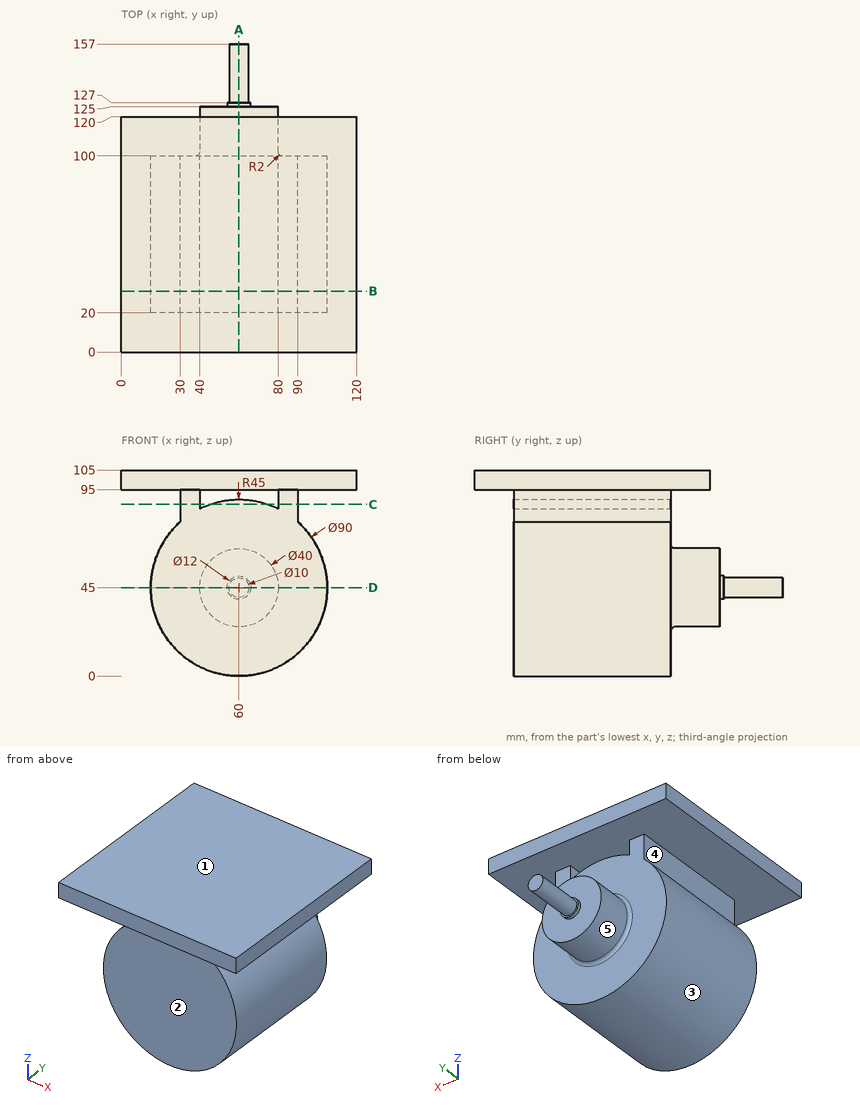
Answer from the drawing. Dimensions are ordinates in mm from the lowest x, y and z of the part. A direction names the side the tool comes from. Give positions to 0.01 mm unless a question says otherwise; leave off trailing zeros. Write each loop counter-clockwise with the first axis right and the second up, starting at its lowest first coordinate (ties: lowest second). Pieces come first, ordered by that corner, then holes. Notation, with made-up numbers: (32.25, -18) - (80.25, -18) arc R11 ccw to (80.25, -9) - close; hole circle Ø2 at (48, -15). An arc over 180 degrees is marked (long way). Answer in a Markdown table with one row per item. Add a question column.
Item 1: Find the intervals of material crossed by L1, parallel to X at y = 88, z = 43.5 (3 decimals); L2, parallel to Z at x = 93.5, y = 11; L3, parallel to Y at x = 30, z = 35.5, in increasing order.
Item 2: Section A-A, the plane x = 60 is taken. Write down the section's boundary in (y, z).
Item 3: Section D-D, the plane z = 45 is taken. Write down the section's boundary in (x, y).
Item 4: Determine the mould class of the marked faces 1, 2 and 3 for opening direction Z: pulls with the +Z half, pulls with the -Z half, needs draft (parallel to the pull), parting line crosses it, or undercut.
Item 5: Section B-B, the plane y = 31 is taken. Write down the section's boundary in (x, z).
Item 6: Flat-ended cylindrical pins translate along their axes: P1, Ø1.5, axis at x = 90.5, y = 74, coming from the -Z side; P2, Ø5, axis at y = 67, z = 90.5, coming from the +X side; P3, Ø1, axis at x = 82.5, z = 16.5, coming from the -Y side. Find the tip coordinate at first contact, or state that the pin passes through.
Item 7: A tool of negligible diameter and unlimited length cuts with its end or side. For the marked faces 4 and 5, from which of +Z, -Z, +X, -X, +Y, -Y can it reach the whole face along a straight path? Write none if from no direction.
Item 8: Section C-C, the plane z = 87.5 is taken. Write down the section's boundary in (x, y).
Recorded:
| question | item | result |
|---|---|---|
| 1 | L1 | x = 15.025 to 104.975 |
| 1 | L2 | z = 95 to 105 |
| 1 | L3 | y = 20 to 100 |
| 2 | outline | (0, 95) - (120, 95) - (120, 105) - (0, 105) - close; (20, 0) - (100, 0) - (100, 23) arc R2 cw to (102, 25) - (125, 25) - (125, 39) - (127, 39) - (127, 40) - (157, 40) - (157, 50) - (127, 50) - (127, 51) - (125, 51) - (125, 65) - (102, 65) arc R2 cw to (100, 67) - (100, 90) - (20, 90) - close |
| 3 | outline | (15, 20) - (105, 20) - (105, 100) - (82, 100) arc R2 cw to (80, 102) - (80, 125) - (66, 125) - (66, 127) - (65, 127) - (65, 157) - (55, 157) - (55, 127) - (54, 127) - (54, 125) - (40, 125) - (40, 102) arc R2 cw to (38, 100) - (15, 100) - close |
| 4 | face 1 | pulls with the +Z half |
| 4 | face 2 | needs draft |
| 4 | face 3 | undercut |
| 5 | outline | (0, 95) - (30, 95) - (30, 78.54) arc R45 ccw (long way) to (90, 78.54) - (90, 95) - (120, 95) - (120, 105) - (0, 105) - close; hole (40, 85.31) arc R45 cw to (80, 85.31) - (80, 95) - (40, 95) - close |
| 6 | P1 | stops at z = 11.24 |
| 6 | P2 | stops at x = 90 |
| 6 | P3 | stops at y = 20 |
| 7 | face 4 | -X, +Y, -Y |
| 7 | face 5 | +Y |
| 8 | outline | (30, 20) - (40, 20) - (40, 100) - (30, 100) - close; (45.21, 20) - (74.79, 20) - (74.79, 100) - (45.21, 100) - close; (80, 20) - (90, 20) - (90, 100) - (80, 100) - close |
